from build123d import *

# Parameters (mm, degrees)
F1_DEPTH = 508
F3_DEPTH = 508


with BuildPart() as f1:
    # F0 (on Front) → F1 (new body)
    with BuildSketch(Plane.XZ):
        Polygon((381, -825.5), (1143, -825.5), (1143, 825.5), (381, 825.5), (381, 190.5), (-381, 190.5), (-381, 825.5), (-1143, 825.5), (-1143, -825.5), (-381, -825.5), align=None)
    extrude(amount=F1_DEPTH)

    # F2 (on face) → F3 (join)
    with BuildSketch(Plane.XZ.offset(508)):
        Polygon((-381, -825.5), (-1143, 825.5), (-1143, -825.5), align=None)
        Polygon((1143, -825.5), (1143, 825.5), (381, -825.5), align=None)
    extrude(amount=F3_DEPTH)


solid = f1.part
Design review of the part built by this model. Coordinates are the model's own, in mm. A direction names the side the tool comes from. Give positions to 0.01 mm unless a question says otherwise; leave off trailing zeros. Write each loop counter-clockwise with the first axis right and the second up, starting at its lowest first coordinate (ties: lowest second). Pieces come first, ordered by that corner, then holes. Notation, with made-up numbers: M -24,56 L -20,56 A27 ccw -20,72 Z; hole C -6.75,27.5 d4. An arc over 180 degrees is marked long. Answer as a JSON object with one key per item and string values. Group by question number.
1) We need section C-C (y = -374.5). Give the boundary of the cut face in (x, z), and give its area (3 significant figures).
2) We need section A-A (z = 455). Give the boundary of the cut face in (x, y), and give its area (3 significant figures).
3) For line 1 along X through (y, z) = (-332, 676.5); line 2 along Z through (x, y) = (255, -250); line 3 along Y through (x, z) = (708, 719.5), list the stretches that pass through material, from the lowest coordinate up.
4) Tool access review of faces 1 (the face through (-16, -501, -825.5)), 2 (the face through (-381, -250, 504)), 3 (the face through (-756.666, -758.444, -11.557)): name each direction out of +Z, -Z, +X, -X, +Y, -Y from which nothing blocks a thin tool from reaching the whole face with its end or side.
5) Clearance check with flat-ended pins moving along their axes: pin 1 Ø6 at (x, y) = (-914, -520.5) entering from +Z; pin 2 Ø2 at (x, z) = (-320, 144) entering from -Y; pin 3 Ø6 at (x, y) = (906, -806) entering from +Z. State where each tip first meets the part, or that it passes through.
6) We need section D-D (z = -670). Give the boundary of the cut face in (x, y).
7) We need section B-B (y = -611). Give the boundary of the cut face in (x, z), and give its area (3 significant figures).
Answer key:
{
 "1": {"outline": "M -1143,-825.5 L 1143,-825.5 L 1143,825.5 L 381,825.5 L 381,190.5 L -381,190.5 L -381,825.5 L -1143,825.5 Z", "area": "3,290,000 mm²"},
 "2": {"outline": "M -1143,-1016 L -972,-1016 L -972,-508 L -381,-508 L -381,0 L -1143,0 Z; M 381,-508 L 972,-508 L 972,-1016 L 1143,-1016 L 1143,0 L 381,0 Z", "area": "948,000 mm²"},
 "3": {"line 1": "x = -1143 to -381, 381 to 1143", "line 2": "z = -825.5 to 190.5", "line 3": "y = -508 to 0"},
 "4": {"face 1": "-Z, +X, -X, +Y, -Y", "face 2": "+Z, +Y, -Y", "face 3": "+Z, -Y"},
 "5": {"pin 1": "stops at z = 335.83", "pin 2": "stops at y = -508", "pin 3": "stops at z = 318.5"},
 "6": {"outline": "M -1143,-1016 L -452.77,-1016 L -452.77,-508 L 452.77,-508 L 452.77,-1016 L 1143,-1016 L 1143,0 L -1143,0 Z"},
 "7": {"outline": "M -1143,-825.5 L -381,-825.5 L -1143,825.5 Z; M 381,-825.5 L 1143,-825.5 L 1143,825.5 Z", "area": "1,260,000 mm²"}
}
